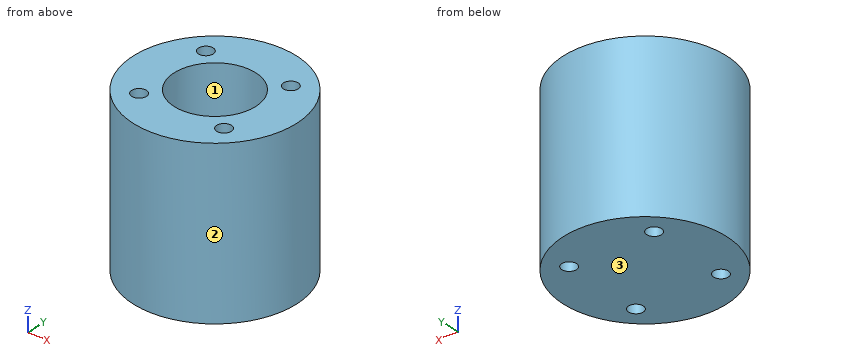
from build123d import *

# Parameters (mm, degrees)
F0_R     = 12.7
F0_R_2   = 1.143
F0_R_3   = 6.35
F1_DEPTH = 25.4
F0_R_4   = 4.0005
F2_DEPTH = 12.7
F3_DEPTH = 7.62


with BuildPart() as f1:
    # F0 (on Top) → F1 (new body)
    with BuildSketch(Plane.XY):
        Circle(F0_R)
        with Locations((-6.593356, -6.437466)):
            Circle(F0_R_2, mode=Mode.SUBTRACT)
        Circle(F0_R_3, mode=Mode.SUBTRACT)
        with Locations((6.593356, -6.437466)):
            Circle(F0_R_2, mode=Mode.SUBTRACT)
        with Locations((-6.593356, 6.437466)):
            Circle(F0_R_2, mode=Mode.SUBTRACT)
        with Locations((6.593356, 6.437466)):
            Circle(F0_R_2, mode=Mode.SUBTRACT)
    extrude(amount=F1_DEPTH)

    # F0 (on Top) → F2 (join)
    with BuildSketch(Plane.XY):
        Circle(F0_R_3)
        Circle(F0_R_4, mode=Mode.SUBTRACT)
    extrude(amount=F2_DEPTH)

    # F0 (on Top) → F3 (join)
    with BuildSketch(Plane.XY):
        Circle(F0_R_4)
    extrude(amount=F3_DEPTH)


solid = f1.part
Part model, mm, in its own coordinate system. Face numbers are marked on the shaded views. Give positions to 0.01 mm unless a question says otherwise; leave off trailing zeros. Write each loop counter-clockwise with the first axis right and the second up, starting at its lowest first coordinate (ties: lowest second). Pieces come first, ordered by that corner, then holes.
1) Probe L1, parallel to X at y = 0.25, z = 10.75; L2, parallel to Y at x = 6.25, z = 4.5; L3, parallel to X at y = 6.5, z = 1.25. List the from-to ranges inside material, lowest first.
Resolved:
L1: x = -12.7 to -3.99, 3.99 to 12.7
L2: y = -11.06 to -7.53, -5.35 to 5.35, 7.53 to 11.06
L3: x = -10.91 to -7.73, -5.45 to 5.45, 7.73 to 10.91
2) Cut at C-C on z = 11. Write the cut outline in (x, y), then the cut area to 3 significant figures.
Resolved:
outline: circle Ø25.4 at (0, 0); hole circle Ø2.29 at (-6.59, -6.44); hole circle Ø2.29 at (-6.59, 6.44); hole circle Ø8 at (0, 0); hole circle Ø2.29 at (6.59, -6.44); hole circle Ø2.29 at (6.59, 6.44)
area: 440 mm2
3) Cut at D-D on x = -7.25. Write the cut outline in (y, z), then the cut area to 3 significant figures.
Resolved:
outline: (-10.43, 0) - (-7.37, 0) - (-7.37, 25.4) - (-10.43, 25.4) - close; (-5.5, 0) - (5.5, 0) - (5.5, 25.4) - (-5.5, 25.4) - close; (7.37, 0) - (10.43, 0) - (10.43, 25.4) - (7.37, 25.4) - close
area: 435 mm2
4) Cut at A-A on x = 0. Write the cut outline in (y, z).
Resolved:
outline: (-12.7, 0) - (12.7, 0) - (12.7, 25.4) - (6.35, 25.4) - (6.35, 12.7) - (4, 12.7) - (4, 7.62) - (-4, 7.62) - (-4, 12.7) - (-6.35, 12.7) - (-6.35, 25.4) - (-12.7, 25.4) - close
5) Pin check, flat tips, straight feed: pin 1 (1.5 mm diameter, centred on y = 4, z = 22.5, fed in from +X); pin 2 (4 mm diameter, centred on x = 1, y = 1, fed in from +Z); pin 3 (4 mm diameter, centred on y = -3, z = 3, fed in from -X). Stop position of each tip, or through.
Resolved:
pin 1: stops at x = 12.28
pin 2: stops at z = 7.62
pin 3: stops at x = -12.66
6) Two-plate mould, pull along Y, no slides. Class the marked faces 1, 2 and 3: released by +Y, released by -Y, zero draft, split by the parting line, or undercut.
Resolved:
face 1: undercut
face 2: split by the parting line
face 3: zero draft
